Can you work these out from the model? Positions are in its coordinate system, mm. A direction names the side the tool comes from. Give positions to 0.01 mm unless a question says otherwise; leave off trailing zeros. Loops run counter-clockwise (first coordinate to the right, second up) from the corner with the lowest first, then second, coordinate; pieces in that order, holes last. Notation, with made-up numbers: M 2,81.25 L 20,81.25 A25 cw 20,117.25 Z; hole C 23,24.5 d6. An arc over 180 degrees is marked long. Use CSV: the item, a comma, the result in double quotes.
from build123d import *

# Parameters (mm, degrees)
SKETCH1_R           = 22.5
BOSS_EXTRUDE1_DEPTH = 12
SKETCH2_R           = 21
CUT_EXTRUDE1_DEPTH  = 10
SKETCH3_R           = 1.5
SKETCH3_R_2         = 7.5
CUT_EXTRUDE2_DEPTH  = 83.0624762


with BuildPart() as part:
    # Sketch1 → Boss-Extrude1 (new body)
    with BuildSketch(Plane.XY):
        Circle(SKETCH1_R)
        with BuildLine():
            Line((-17, -14.739402973), (-17, -78))
            Line((-17, -78), (17, -78))
            Line((17, -78), (17, -14.739402973))
            ThreePointArc((17, -14.739402973), (0, -22.5), (-17, -14.739402973))
        make_face()
    extrude(amount=BOSS_EXTRUDE1_DEPTH)

    # Sketch2 → Cut-Extrude1 (cut)
    with BuildSketch(Plane(origin=(0, 0, 0), x_dir=(-1, 0, 0), z_dir=(0, 0, -1))):
        Circle(SKETCH2_R)
    extrude(amount=-CUT_EXTRUDE1_DEPTH, mode=Mode.SUBTRACT)

    # Sketch3 → Cut-Extrude2 (cut, through all)
    with BuildSketch(Plane.XY.offset(12)):
        with Locations((0, 15)):
            Circle(SKETCH3_R)
        with Locations((12.990381057, -7.5)):
            Circle(SKETCH3_R)
        with Locations((-12.990381057, -7.5)):
            Circle(SKETCH3_R)
        Circle(SKETCH3_R_2)
    extrude(amount=-CUT_EXTRUDE2_DEPTH, mode=Mode.SUBTRACT)


solid = part.part
Q1. If we mould it in two halves opening along X, with no side actions, what happens to faces 1 (the flat face through (17, -47, 6)), 2 (the cylindrical face through (-20.03, 6.31, 4.93)), 3 (the flat face through (0, -27, 12))? For each: released by +X, released by -X, zero draft, split by the parting line, or undercut.
Model answer:
face 1,"released by +X"
face 2,"undercut"
face 3,"zero draft"
Q2. For faces 4 (the flat face through (0, -9, 10)), 5 (the cylindrical face through (-7.493, 0.33, 11.014)), 6 (the flat face through (-17, -46, 6)), which set-ups out of +Z, -Z, +X, -X, +Y, -Y let a thin tool reach every point of the face, with its end or its side?
Model answer:
face 4,"-Z"
face 5,"+Z, -Z"
face 6,"+Z, -Z, -X, -Y"
Q3. I'm going to push flat-ended pins straight in: P1, Ø9, axis at x = 0, y = 0, coming from the +Z side; P2, Ø3.5, axis at x = 12.99, y = -7.5, coming from the +Z side; P3, Ø3, axis at x = -7, y = 10.5, coming from the -Z side; P4, Ø6, axis at y = -34, z = 5.5, coming from the +X side. Where does each tip first touch, or does it pass through?
Model answer:
P1,"through"
P2,"z = 12"
P3,"z = 10"
P4,"x = 17"
Q4. Please list where these lines run through material, in increasing order: L1, parallel to Y at x = 0, z = 2.75; L2, parallel to X at y = -42.5, z = 2.5; L3, parallel to Z at x = -1, y = -15.5. Write a range as from..to.
Model answer:
L1,"-78..-21, 21..22.5"
L2,"-17..17"
L3,"10..12"
Q5. I want a section at C-C, the plane z = 8. Please give me the cut outline in (x, y), then the cut area to 3 significant figures.
Model answer:
outline,"M -17,-78 L 17,-78 L 17,-14.74 A22.5 ccw long -17,-14.74 Z; hole C 0,0 d42"
area,"2,170 mm2"
Q6. I want a section at A-A, the plane y = 0. Please give me the cut outline in (x, z).
Model answer:
outline,"M -22.5,0 L -21,0 L -21,10 L -7.5,10 L -7.5,12 L -22.5,12 Z; M 7.5,10 L 21,10 L 21,0 L 22.5,0 L 22.5,12 L 7.5,12 Z"
Q7. I want a section at B-B, the plane x = 4. Please give me the cut outline in (y, z), then the cut area to 3 significant figures.
Model answer:
outline,"M -78,0 L -20.62,0 L -20.62,10 L -6.34,10 L -6.34,12 L -78,12 Z; M 6.34,10 L 20.62,10 L 20.62,0 L 22.14,0 L 22.14,12 L 6.34,12 Z"
area,"764 mm2"
Q8. I want a section at D-D, the plane x = 19.5. Please give me the cut outline in (y, z), then the cut area to 3 significant figures.
Model answer:
outline,"M -11.22,0 L -7.79,0 L -7.79,10 L 7.79,10 L 7.79,0 L 11.22,0 L 11.22,12 L -11.22,12 Z"
area,"114 mm2"
